Part model, mm, in its own coordinate system. A direction names the side the tool comes from. Round coordinates to 2 decimals unless told otherwise and drop trailing zeros. Order: outer loops, then holes, each group sorted by start corner. A loop starts at its lowest first (then second) coordinate and runs counter-clockwise, first axis right, second up. Notation, with made-up numbers: (27.25, 73.25) - (48.25, 73.25) arc R29 ccw to (48.25, 100.25) - close; hole circle Ø3 at (65.5, 31.25). An arc over 180 degrees is marked (long way). Return JSON: item names as keys, results as strings. Group by question number.
Item 1: Saw through at C-C on z = 3.5. List the corners of the cut face in (x, y).
Item 2: Drop flat-ended pins along their axis: pin 1 (4 mm diameter, centred on y = 2.5, z = -21, fed in from +X); pin 2 (4 mm diameter, centred on x = 8.5, z = -10.5, fed in from -Y); pin 3 (3 mm diameter, centred on y = -8, z = -15, fed in from -X). Give the stop position or say it passes through.
Item 3: Two-plate mould, pull along X, no slides. Class faces 3 (the face through (10, 0, -28)), 4 (the face through (0, 0, 0)), 5 (the face through (7.5, 0, -14)), 6 (the face through (-14, 0, -11)): released by +X, released by -X, zero draft, split by the parting line, or undercut.
Item 4: Tool access for faces 1 (the face through (-7.5, 0, -14)), 2 (the face through (0, -11.822, 2)): list every direction of +Z, -Z, +X, -X, +Y, -Y with a clear straight run to the whole face (end or side of a thin tool).
Item 5: Saw through at D-D on x = 5.5. List the corners of the cut face in (y, z), and give its area (3 significant figures).
Item 6: Saw through at B-B on y = 8.25. List the corners of the cut face in (x, z), and give its area (3 significant figures).
Item 7: Saw through at A-A on z = -18.5. List the corners of the cut face in (x, y), and give its area (3 significant figures).
Item 8: Probe probe 1 along Z at (x, y) = (-4, -3.25); probe 2 along X at (y, z) = (-2.75, -14); probe 3 along X at (y, z) = (6, -5.5). List the from-to ranges inside material, lowest first.
```python
from build123d import *

# Parameters (mm, degrees)
F1_DEPTH = 5
F2_DEPTH = 28


with BuildPart() as f1:
    # F0 (on Top) → F1 (new body)
    with BuildSketch(Plane.XY):
        with BuildLine():
            Line((-7.5, 0), (-7.5, 11.82159))
            ThreePointArc((-7.5, 11.82159), (-14, 0), (-7.5, -11.82159))
            Line((-7.5, -11.82159), (-7.5, 0))
        make_face()
        with BuildLine():
            Line((-7.5, -11.82159), (7.5, -11.82159))
            Line((7.5, -11.82159), (7.5, 0))
            Line((7.5, 0), (5, 0))
            ThreePointArc((5, 0), (0, -5), (-5, 0))
            Line((-5, 0), (-7.5, 0))
            Line((-7.5, 0), (-7.5, -11.82159))
        make_face()
        with BuildLine():
            Line((7.5, 0), (7.5, 11.82159))
            Line((7.5, 11.82159), (-7.5, 11.82159))
            Line((-7.5, 11.82159), (-7.5, 0))
            Line((-7.5, 0), (-5, 0))
            ThreePointArc((-5, 0), (0, 5), (5, 0))
            Line((5, 0), (7.5, 0))
        make_face()
        with BuildLine():
            ThreePointArc((7.5, -11.82159), (12.267844, -6.745369), (14, 0))
            ThreePointArc((14, 0), (12.267844, 6.745369), (7.5, 11.82159))
            Line((7.5, 11.82159), (7.5, 0))
            Line((7.5, 0), (7.5, -11.82159))
        make_face()
        with BuildLine():
            Line((0, 0), (5, 0))
            ThreePointArc((5, 0), (0, 5), (-5, 0))
            Line((-5, 0), (0, 0))
        make_face()
        with BuildLine():
            ThreePointArc((-5, 0), (0, -5), (5, 0))
            Line((5, 0), (0, 0))
            Line((0, 0), (-5, 0))
        make_face()
    extrude(amount=F1_DEPTH)

    # F0 (on Top) → F2 (join)
    with BuildSketch(Plane.XY):
        with BuildLine():
            Line((-7.5, 0), (-7.5, 11.82159))
            ThreePointArc((-7.5, 11.82159), (-14, 0), (-7.5, -11.82159))
            Line((-7.5, -11.82159), (-7.5, 0))
        make_face()
        with BuildLine():
            ThreePointArc((7.5, -11.82159), (12.267844, -6.745369), (14, 0))
            ThreePointArc((14, 0), (12.267844, 6.745369), (7.5, 11.82159))
            Line((7.5, 11.82159), (7.5, 0))
            Line((7.5, 0), (7.5, -11.82159))
        make_face()
    extrude(amount=-F2_DEPTH)


solid = f1.part
```
Filled in:
{
 "1": {"outline": "(-7.5, -11.82) - (7.5, -11.82) arc R14 ccw to (7.5, 11.82) - (-7.5, 11.82) arc R14 ccw to start"},
 "2": {"pin 1": "stops at x = 13.99", "pin 2": "stops at y = -11.82", "pin 3": "stops at x = -12.4"},
 "3": {"face 3": "zero draft", "face 4": "undercut", "face 5": "undercut", "face 6": "released by -X"},
 "4": {"face 1": "-Z, +Y, -Y", "face 2": "+Z, -Z, +X, -X, -Y"},
 "5": {"outline": "(-11.82, 0) - (11.82, 0) - (11.82, 5) - (-11.82, 5) - close", "area": "118 mm^2"},
 "6": {"outline": "(-11.31, -28) - (-7.5, -28) - (-7.5, 0) - (7.5, 0) - (7.5, -28) - (11.31, -28) - (11.31, 5) - (-11.31, 5) - close", "area": "327 mm^2"},
 "7": {"outline": "(-7.5, -11.82) - (-7.5, 11.82) arc R14 ccw to start; (7.5, -11.82) arc R14 ccw to (7.5, 11.82) - close", "area": "217 mm^2"},
 "8": {"probe 1": "z = 0 to 5", "probe 2": "x = -13.73 to -7.5, 7.5 to 13.73", "probe 3": "x = -12.65 to -7.5, 7.5 to 12.65"}
}
